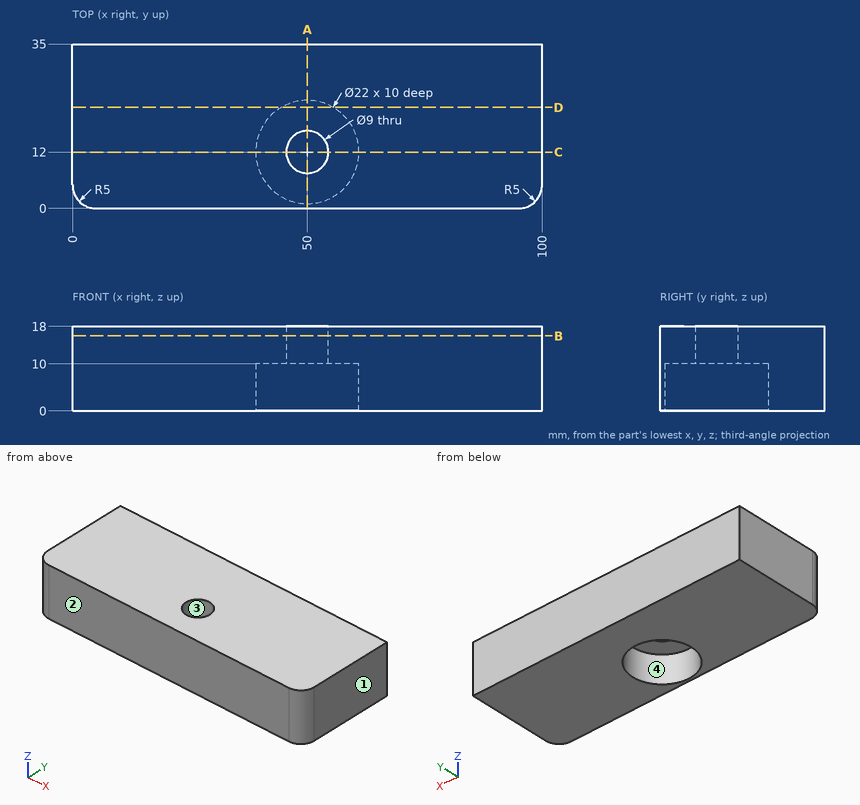
Design review of the part shown in the three views and the two pictorial views. Dimensions are in mm from the part's minimum x, y and z. Coordinates: 2 decimals unless noted, no trailing zeros. Loops run counter-clockwise (first coordinate to the right, second up) from the corner with the lowest first, then second, coordinate; pieces in that order, holes last. Notation, with made-up numbers: (83.5, 85.25) - (94.5, 85.25) arc R17 cw to (94.5, 95.25) - close; hole circle Ø11 at (82.5, 31.5). An arc over 180 degrees is marked (long way). Use a Markdown table: item, result. Add a question column.
Item 1: We need section C-C (y = 12). Give the boundary of the cut face in (x, z), and give its area (3 significant figures).
Item 2: Mouldability with a two-part tool opening along X and no side actions: class the marked faces 1, 2, 3 and 4 as pulls with the +X half, pulls with the -X half, needs draft (parallel to the pull), parting line crosses it, or undercut.
Item 3: Insertion check: pin 1 Ø13 at (x, y) = (50, 12) entering from -Z. The pin has a flat end and moves straight along its axis. Give the tip position at first contact, or say it passes through.
Item 4: We need section B-B (z = 16). Give the boundary of the cut face in (x, y).
Item 5: We need section D-D (y = 21.5). Give the boundary of the cut face in (x, z).
Item 6: We need section A-A (x = 50). Give the boundary of the cut face in (y, z).
Item 7: For line 1 (Y direction, x = 50, z = 3.5); line 2 (Y direction, x = 50, z = 14.5); line 3 (Z direction, x = 59, y = 15), list the stretches that pass through material, from the lowest coordinate up.
Results list:
| question | item | result |
|---|---|---|
| 1 | outline | (0, 0) - (39, 0) - (39, 10) - (45.5, 10) - (45.5, 18) - (0, 18) - close; (54.5, 10) - (61, 10) - (61, 0) - (100, 0) - (100, 18) - (54.5, 18) - close |
| 1 | area | 1,510 mm^2 |
| 2 | face 1 | pulls with the +X half |
| 2 | face 2 | needs draft |
| 2 | face 3 | undercut |
| 2 | face 4 | undercut |
| 3 | pin 1 | stops at z = 10 |
| 4 | outline | (0, 5) arc R5 ccw to (5, 0) - (95, 0) arc R5 ccw to (100, 5) - (100, 35) - (0, 35) - close; hole circle Ø9 at (50, 12) |
| 5 | outline | (0, 0) - (44.45, 0) - (44.45, 10) - (55.55, 10) - (55.55, 0) - (100, 0) - (100, 18) - (0, 18) - close |
| 6 | outline | (0, 0) - (1, 0) - (1, 10) - (7.5, 10) - (7.5, 18) - (0, 18) - close; (16.5, 10) - (23, 10) - (23, 0) - (35, 0) - (35, 18) - (16.5, 18) - close |
| 7 | line 1 | y = 0 to 1, 23 to 35 |
| 7 | line 2 | y = 0 to 7.5, 16.5 to 35 |
| 7 | line 3 | z = 10 to 18 |
